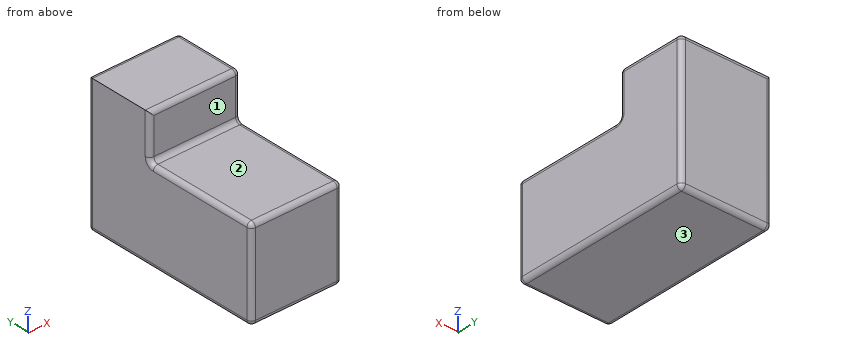
Solid Edge part; units mm, degrees
sketch "Sketch1" plane through (0, 0, 0) normal (0, 0, 1) x (1, 0, 0)
  line L0 (-2, -4) -> (2, -4)
  line L1 (2, -4) -> (2, 4)
  line L2 (2, 4) -> (-2, 4)
  line L3 (-2, 4) -> (-2, -4)
  dimension "D1" = 2
  dimension "D2" = 2
extrude "Protrusion1" add sketch "Sketch1" along normal blind 4
sketch "Sketch2" plane through (0, 0, 4) normal (0, 0, 1) x (1, 0, 0)
  line L0 (-2, 4) -> (2, 4)
  line L1 (2, 4) -> (2, 1)
  line L2 (2, 1) -> (-2, 1)
  line L3 (-2, 1) -> (-2, 4)
extrude "ExtrudedProtrusion_2" add sketch "Sketch2" along normal blind 2
fillet "Round_1" radius 0.2 17 edges at (0, 1, 6) (0, 1, 4) (2, 2.5, 6) (0, 4, 6) (2, 4, 3) (2, -1.5, 4) (-2, -1.5, 4) (0, -4, 4) (0, -4, 0) (2, 0, 0) (-2, 0, 0) (-2, 4, 3) (0, 4, 0) (-2, -4, 2) (2, -4, 2) (2, 1, 5) (-2, 1, 5)
properties material "Steel"
Verification items for the finished model (mm, model axes). Face numbers are marked on the shaded views. Give positions to 0.01 mm unless a question says otherwise; leave off trailing zeros. Loops run counter-clockwise (first coordinate to the right, second up) from the corner with the lowest first, then second, coordinate; pieces in that order, holes last.
1) Sectioned sample at B-B, the plane y = -2. Enter the section's corners in (x, z), then the cut area to 3 significant figures.
2) Draft check along Z on the marked faces 1, 2 and 3. Enter one of: pulls with the +Z half, pulls with the -Z half, needs draft (parallel to the pull), parting line crosses it, or undercut.
3) Thickness scan on line 1 along Z through (x, y) = (1.6, -1); line 2 along Y through (x, z) = (-0.05, 5.5). Record the ranges inside material, lowest first.
4) Sectioned sample at A-A, the plane x = -1.35. Enter the section's corners in (y, z), then the cut area to 3 significant figures.
5) Sectioned sample at C-C, the plane z = 5.5. Enter the section's corners in (x, y), then the cut area to 3 significant figures.
6) Depth check by flat-ended pin: pin 1 Ø1.8 at (x, y) = (0, -2) entering from +Z; pin 2 Ø0.8 at (x, z) = (-1, 5) entering from -Y. Enter the tip coordinate at first touch or a pass-through.
Answers:
1. outline: (-2, 0.2) arc R0.2 ccw to (-1.8, 0) - (1.8, 0) arc R0.2 ccw to (2, 0.2) - (2, 3.8) arc R0.2 ccw to (1.8, 4) - (-1.8, 4) arc R0.2 ccw to (-2, 3.8) - close
1. area: 16.0 mm2
2. face 1: needs draft
2. face 2: pulls with the +Z half
2. face 3: pulls with the -Z half
3. line 1: z = 0 to 4
3. line 2: y = 1 to 4
4. outline: (-4, 0.2) arc R0.2 ccw to (-3.8, 0) - (3.8, 0) arc R0.2 ccw to (4, 0.2) - (4, 5.8) arc R0.2 ccw to (3.8, 6) - (1.2, 6) arc R0.2 ccw to (1, 5.8) - (1, 4.2) arc R0.2 cw to (0.8, 4) - (-3.8, 4) arc R0.2 ccw to (-4, 3.8) - close
4. area: 38.0 mm2
5. outline: (-2, 1.2) arc R0.2 ccw to (-1.8, 1) - (1.8, 1) arc R0.2 ccw to (2, 1.2) - (2, 3.8) arc R0.2 ccw to (1.8, 4) - (-1.8, 4) arc R0.2 ccw to (-2, 3.8) - close
5. area: 12.0 mm2
6. pin 1: stops at z = 4
6. pin 2: stops at y = 1
